The model under review builds one solid part; all positions refer to its coordinate system, in mm. Give positions to 0.01 mm unless a question says otherwise; leave off trailing zeros. Order: outer loops, then holes, each group sorted by start corner. A loop starts at its lowest first (then second) coordinate and runs counter-clockwise, first axis right, second up. Notation, with made-up numbers: (70.25, -36) - (75.25, -36) arc R15 cw to (75.25, -30) - close; hole circle Ø8 at (86.25, -37.75). An arc over 180 degrees is marked (long way). Use a Markdown table: item, result. Add a question column.
```python
from build123d import *

# Parameters (mm, degrees)
F0_R     = 2.5
F0_R_2   = 1.5
F0_R_3   = 11
F0_R_4   = 3
F1_DEPTH = 3


with BuildPart() as f1:
    # F0 (on Top) → F1 (new body)
    with BuildSketch(Plane.XY):
        with BuildLine():
            Line((-48.422295, -70.076307), (29.060322, -70.076307))
            ThreePointArc((29.060322, -70.076307), (32.595856, -68.611841), (34.060322, -65.076307))
            Line((34.060322, -65.076307), (34.060322, 14.923693))
            ThreePointArc((34.060322, 14.923693), (32.595856, 18.459226), (29.060322, 19.923693))
            Line((29.060322, 19.923693), (0, 98.959506))
            Line((0, 98.959506), (-18.166697, 98.959506))
            Line((-18.166697, 98.959506), (-48.422295, 19.923693))
            ThreePointArc((-48.422295, 19.923693), (-51.957828, 18.459226), (-53.422295, 14.923693))
            Line((-53.422295, 14.923693), (-53.422295, -65.076307))
            ThreePointArc((-53.422295, -65.076307), (-51.957828, -68.611841), (-48.422295, -70.076307))
        make_face()
        with Locations((-32.677192, -64.076307)):
            Circle(F0_R, mode=Mode.SUBTRACT)
        with Locations((-45.05799, -6.326307)):
            Circle(F0_R, mode=Mode.SUBTRACT)
        with Locations((-24.306103, 2.083096)):
            Circle(F0_R_2, mode=Mode.SUBTRACT)
        with Locations((17.322808, -64.076307)):
            Circle(F0_R, mode=Mode.SUBTRACT)
        with Locations((6.693897, 2.083096)):
            Circle(F0_R_2, mode=Mode.SUBTRACT)
        with Locations((24.94201, -6.326307)):
            Circle(F0_R, mode=Mode.SUBTRACT)
        with Locations((-24.306103, 33.083096)):
            Circle(F0_R_2, mode=Mode.SUBTRACT)
        with Locations((-8.806103, 17.583096)):
            Circle(F0_R_3, mode=Mode.SUBTRACT)
        with Locations((6.693897, 33.083096)):
            Circle(F0_R_2, mode=Mode.SUBTRACT)
        with Locations((-8.806103, 63.673693)):
            Circle(F0_R_4, mode=Mode.SUBTRACT)
        with Locations((-8.806103, 83.673693)):
            Circle(F0_R_4, mode=Mode.SUBTRACT)
    extrude(amount=F1_DEPTH)


solid = f1.part
```
Q1. We need section C-C (x = -33). Write out the cut boundary in (y, z), plus the area to 3 significant figures.
Q2. We need section B-B (y = 26). Write out the cut boundary in (x, z), plus the area to 3 significant figures.
Q3. We need section A-A (z = 0.65). Count the separate pieces of the cut face and the enclosed holes in it, plus the area to 3 significant figures.
Q4. Wall thickness on probe 1 along X at (y, z) = (24.5, 0.9); probe 2 along Y at (x, z) = (-13.5, 2.7); probe 3 along Y at (x, z) = (-48.5, 0.3): over which ranges is each line inside the solid? List them lowest first.
Q5. We need section D-D (x = -10). Write out the cut boundary in (y, z).
Q6. Draft analysis for pull direction Y (two halves, no side actions). For faces 1 (the flat face through (34.06, -26, 1)), 2 (the cylindrical face through (33, 18, 1)), 3 (the cylindrical face through (-9.456, 60.745, 1.479)), 4 (the cylindrical face through (5.59, 3.1, 1.48)), state which applies: pulls with the +Y half, pulls with the -Y half, needs draft (parallel to the pull), parting line crosses it, or undercut.
Here are the results:
| question | item | result |
|---|---|---|
| 1 | outline | (-70.08, 0) - (-66.56, 0) - (-66.56, 3) - (-70.08, 3) - close; (-61.6, 0) - (60.21, 0) - (60.21, 3) - (-61.6, 3) - close |
| 1 | area | 376 mm2 |
| 2 | outline | (-46.1, 0) - (-15.89, 0) - (-15.89, 3) - (-46.1, 3) - close; (-1.72, 0) - (26.83, 0) - (26.83, 3) - (-1.72, 3) - close |
| 2 | area | 176 mm2 |
| 3 | separate pieces | 1 |
| 3 | enclosed holes | 11 |
| 3 | area | 11,100 mm2 |
| 4 | probe 1 | -46.67 to -17.36, -0.25 to 27.38 |
| 4 | probe 2 | -70.08 to 7.63, 27.53 to 98.96 |
| 4 | probe 3 | -70.08 to 19.92 |
| 5 | outline | (-70.08, 0) - (6.65, 0) - (6.65, 3) - (-70.08, 3) - close; (28.52, 0) - (60.92, 0) - (60.92, 3) - (28.52, 3) - close; (66.43, 0) - (80.92, 0) - (80.92, 3) - (66.43, 3) - close; (86.43, 0) - (98.96, 0) - (98.96, 3) - (86.43, 3) - close |
| 6 | face 1 | needs draft |
| 6 | face 2 | pulls with the +Y half |
| 6 | face 3 | undercut |
| 6 | face 4 | undercut |
